Autodesk Inventor part; units mm, degrees
ref_plane "YZ Plane" through (0, 0, 0) normal (1, 0, 0) x (0, 1, 0)
ref_plane "XZ Plane" through (0, 0, 0) normal (0, 1, 0) x (-1, 0, 0)
ref_plane "XY Plane" through (0, 0, 0) normal (0, 0, 1) x (1, 0, 0)
sketch "Sketch1" plane through (0, 0, 0) normal (0, 0, 1) x (1, 0, 0)
  line L0 (0, 0) -> (27, 0)
  line L1 (27, 0) -> (27, 10)
  line L2 (27, 10) -> (0, 10)
  line L3 (0, 10) -> (0, 0)
  dimension "d0" = 27
  dimension "d1" = 10
extrude "Extrusion1" add sketch "Sketch1" along normal blind 16
fillet "Fillet1" radius 8 2 edges at (27, 5, 16) (27, 5, 0)
sketch "Sketch2" plane through (0, 10, 16) normal (0, 1, 0) x (1, 0, 0)
  circle A0 centre (19, 8) radius 5.05
  arc A1 (19, 0) -> (19, 16) centre (19, 8) ccw
  point P0 (0, 16)
  dimension "d5" = 10.1
extrude "Extrusion2" cut sketch "Sketch2" against normal through all
sketch "Sketch3" plane through (0, 0, 0) normal (-1, 0, 0) x (0, 0, 1)
  line L0 (0, 0) -> (16, 10) construction
  point P0 (8, 5)
  point P1 (8, 5)
hole "Hole1" at (0, 5, 8) direction (1, 0, 0) diameter 4.917 depth 12 tip angle 118
sketch "Sketch4" plane through (0, 0, 0) normal (-1, 0, 0) x (0, 0, 1)
  line L0 (0, 0) -> (16, 0)
  arc A0 (15.1987, 0) -> (15.1987, 10) centre (0, 5) ccw
  line L1 (0, 10) -> (16, 10)
  line L2 (16, 10) -> (16, 0)
  point P0 (16, 5)
  dimension "d15" = 16
sketch3d "3D Sketch1"
  line L0 (0, 10, 16) -> (19, 10, 16)
  arc A0 (19, 10, 0) -> (24.6569, 10, 2.3431) centre (19, 10, 8) ccw
  arc A1 (24.6569, 10, 2.3431) -> (27, 10, 8) centre (19, 10, 8) ccw
  arc A2 (27, 10, 8) -> (24.6569, 10, 13.6569) centre (19, 10, 8) ccw
  arc A3 (24.6569, 10, 13.6569) -> (19, 10, 16) centre (19, 10, 8) ccw
  line L1 (19, 10, 0) -> (0, 10, 0)
sweep "Sweep1" cut profiles "Sketch4" path "3D Sketch1"
chamfer "Chamfer1" distance 1 angle 45 3 edges at (13.95, 10, 8) (13.95, 0, 8) (0, 5, 5.5415)
properties part number "GMW-6-1 eye M6x1" material "Steel, Alloy"
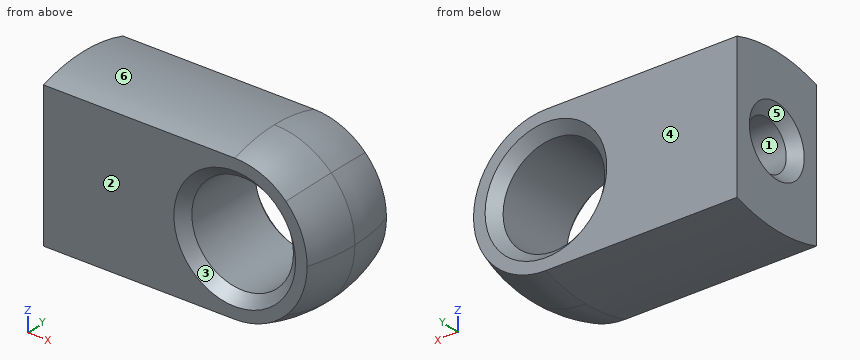
Could you check a few things on this model? Use its own coordinates, in mm. Face numbers are marked on the shaded views. A direction names the side the tool comes from. Give positions to 0.01 mm unless a question says otherwise; leave off trailing zeros. Write each loop counter-clockwise with the first axis right and the second up, starting at its lowest first coordinate (ties: lowest second). Pieces come first, ordered by that corner, then holes. Notation, with made-up numbers: (-20, 29) -> (-2, 29) arc R28 cw to (-2, 49) -> close; hole circle Ø3 at (87.25, -1.75). An arc over 180 degrees is marked (long way). Answer as CSV lines item,"result". Start each with the question number.
(1) I'm going to push flat-ended pins straight in: pin 1 Ø2 at (y, z) = (6.5, 12.5) entering from +X; pin 2 Ø6 at (y, z) = (7, 12.5) entering from +X. Where does each tip first touch, or does it pass through?
(2) If we section it at A-A, the plane x = 8: Write out the boundary of the cut face in (y, z).
(3) Which directions (+Z, -Z, +X, -X, +Y, -Y) give clear straight access to the entire face, cutting with the end or side of a thin tool? Please do the marked faces 1 and 2.
(4) Please list where these lines run through material, in increasing order: line 1 (Z direction, x = 8.25, y = 5); line 2 (Z direction, x = 19, y = 5.25); line 3 (Y direction, x = 4, z = 8).
(5) If we mould it in two halves opening along Z, with no side actions, what happens to the marked faces 3, 4, 5 and 6? For each: +Z half, -Z half, draft (parallel to the pull), parting line (faces both ways), or undercut.
Answer list:
1,pin 1,"x = 26.13"
1,pin 2,"x = 26.79"
2,outline,"(0, 0.8) arc R16 ccw to (10, 0.8) -> (10, 15.2) arc R16 ccw to (0, 15.2) -> close; hole circle Ø4.92 at (5, 8)"
3,face 1,"-X"
3,face 2,"+Z, -Z, +X, -X, -Y"
4,line 1,"0 to 5.54, 10.46 to 16"
4,line 2,"0 to 2.95, 13.05 to 16"
4,line 3,"0 to 2.54, 7.46 to 10"
5,face 3,"undercut"
5,face 4,"draft"
5,face 5,"undercut"
5,face 6,"+Z half"
